from build123d import *

# Parameters (mm, degrees)
SKETCH1_W           = 20
SKETCH1_H           = 130
SKETCH1_R           = 2.5
BOSS_EXTRUDE1_DEPTH = 60
BOSS_EXTRUDE2_DEPTH = 130
CUT_EXTRUDE2_DEPTH  = 156.241746963
CUT_EXTRUDE3_DEPTH  = 25
SKETCH5_R           = 10
CUT_EXTRUDE4_DEPTH  = 147.694623422
SKETCH6_R           = 6
CUT_EXTRUDE8_DEPTH  = 55
SKETCH7_R           = 2.5
CUT_EXTRUDE9_DEPTH  = 5
SKETCH9_R           = 6
CUT_EXTRUDE10_DEPTH = 151.423561372


with BuildPart() as part:
    # Sketch1 → Boss-Extrude1 (new body)
    with BuildSketch(Plane.XY):
        with Locations((0, 65)):
            Rectangle(SKETCH1_W, SKETCH1_H)
        with Locations((0, 119.20647252)):
            Circle(SKETCH1_R, mode=Mode.SUBTRACT)
        with Locations((0, 68.70647252)):
            Circle(SKETCH1_R, mode=Mode.SUBTRACT)
    extrude(amount=BOSS_EXTRUDE1_DEPTH)

    # Sketch2 → Boss-Extrude2 (add)
    with BuildSketch(Plane(origin=(0, 130, 0), x_dir=(1, 0, 0), z_dir=(0, 1, 0))):
        Polygon((10, 0), (60, -50), (60, -60), (10, -60), align=None)
    extrude(amount=-BOSS_EXTRUDE2_DEPTH)

    # Sketch4 → Cut-Extrude2 (cut, through all)
    with BuildSketch(Plane(origin=(0, 0, 0), x_dir=(-1, 0, 0), z_dir=(0, 0, -1))):
        with BuildLine():
            ThreePointArc((-1.666666667, 129.066605492), (6.454972244, 126.844098678), (10, 119.20647252))
            Line((10, 119.20647252), (10, 130))
            Line((10, 130), (-10, 130))
            Line((-10, 130), (-10, 127.658015067))
            Line((-10, 127.658015067), (-1.666666667, 129.066605492))
        make_face()
        Polygon((-60, 130), (-60, 119.20647252), (-10, 127.658015067), (-10, 130), align=None)
    extrude(amount=-CUT_EXTRUDE2_DEPTH, mode=Mode.SUBTRACT)

    # Sketch4<5> → Cut-Extrude3 (cut)
    with BuildSketch(Plane(origin=(0, 0, 0), x_dir=(-1, 0, 0), z_dir=(0, 0, -1))):
        with BuildLine():
            Line((10, 0), (10, 68.70647252))
            ThreePointArc((10, 68.70647252), (6.454972244, 61.068846362), (-1.666666667, 58.846339548))
            Line((-1.666666667, 58.846339548), (-10, 60.254929973))
            Line((-10, 60.254929973), (-10, 0))
            Line((-10, 0), (10, 0))
        make_face()
        Polygon((-10, 60.254929973), (-60, 68.70647252), (-60, 0), (-10, 0), align=None)
    extrude(amount=-CUT_EXTRUDE3_DEPTH, mode=Mode.SUBTRACT)

    # Sketch5 → Cut-Extrude4 (cut, through all)
    with BuildSketch(Plane(origin=(0, 0, 25), x_dir=(-1, 0, 0), z_dir=(0, 0, -1))):
        with Locations((10, 0)):
            Circle(SKETCH5_R)
    extrude(amount=-CUT_EXTRUDE4_DEPTH, mode=Mode.SUBTRACT)

    # Sketch6 → Cut-Extrude8 (cut)
    with BuildSketch(Plane.XY.offset(60)):
        with Locations((0, 119.20647252)):
            Circle(SKETCH6_R)
        with Locations((0, 68.70647252)):
            Circle(SKETCH6_R)
    extrude(amount=-CUT_EXTRUDE8_DEPTH, mode=Mode.SUBTRACT)

    # Sketch7 → Cut-Extrude9 (cut)
    with BuildSketch(Plane.XZ):
        with Locations(Location((10, 50, 0), (0, 0, 270))):
            Circle(SKETCH7_R)
        with Locations(Location((40, 50, 0), (0, 0, 270))):
            Circle(SKETCH7_R)
        with Locations(Location((25, 35, 0), (0, 0, 270))):
            Circle(SKETCH7_R)
    extrude(amount=-CUT_EXTRUDE9_DEPTH, mode=Mode.SUBTRACT)

    # Sketch9 → Cut-Extrude10 (cut, through all)
    with BuildSketch(Plane.XZ.offset(-5)):
        with Locations(Location((10, 50, 0), (0, 0, 270))):
            Circle(SKETCH9_R)
        with Locations(Location((25, 35, 0), (0, 0, 270))):
            Circle(SKETCH9_R)
        with Locations(Location((40, 50, 0), (0, 0, 270))):
            Circle(SKETCH9_R)
    extrude(amount=-CUT_EXTRUDE10_DEPTH, mode=Mode.SUBTRACT)


solid = part.part
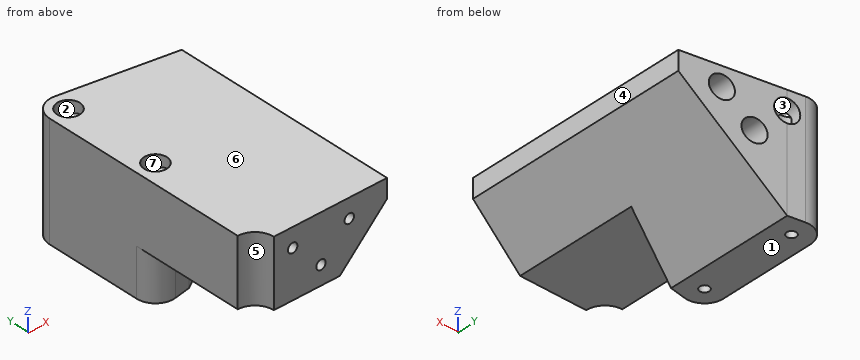
Source: CAD feature listing. Evaluate the final solid. Frame: model axes, mm. Face numbers are marked on the shaded views. A direction names the side the tool comes from. Give positions to 0.01 mm unless a question says otherwise; leave off trailing zeros. Order: outer loops, then holes, each group sorted by start corner. A loop starts at its lowest first (then second) coordinate and runs counter-clockwise, first axis right, second up. Notation, with made-up numbers: (83.5, 23.25) -> (112.5, 23.25) arc R3 ccw to (112.5, 28.25) -> close; hole circle Ø3 at (-34, -39). An arc over 180 degrees is marked (long way). Write item = value, one per line.
Q1. Cut plane C-C, the plane z = 27.5. Output: boundary loops of the cut face in (x, y), and give its area (3 significant figures).
Data:
outline = (-10, 10) arc R10 cw to (0, 0) -> (37.5, 0) -> (37.5, 123.01) -> (1.67, 129.07) arc R10 ccw to (-10, 119.21) -> close; hole circle Ø12 at (0, 68.71); hole circle Ø12 at (0, 119.21)
area = 5,700 mm^2
Q2. Pin query (flat end, axial travel): pin 1 (6.5 mm diameter, centred on x = 0, y = 68.71, fed in from +Z); pin 2 (6 mm diameter, centred on x = 25.5, z = 35, fed in from +Y); pin 3 (2 mm diameter, centred on x = 2, z = 19.5, fed in from -Y). Return the tip coordinate at first contact, or that it passes through.
Data:
pin_1 = 5
pin_2 = 5
pin_3 = 58.76
Q3. Cut plane D-D, the plane z = 35. Output: boundary loops of the cut face in (x, y).
Data:
outline = (-10, 10) arc R10 cw to (0, 0) -> (22.5, 0) -> (22.5, 5) -> (19, 5) -> (19, 126.14) -> (1.67, 129.07) arc R10 ccw to (-10, 119.21) -> close; (27.5, 0) -> (45, 0) -> (45, 121.74) -> (31, 124.11) -> (31, 5) -> (27.5, 5) -> close; hole circle Ø12 at (0, 68.71); hole circle Ø12 at (0, 119.21)
Q4. Material intervals for line 1 (Y direction, x = 0, z = 3.65); line 2 (X direction, y = 54, z = 50); line 3 (Y direction, x = -2, z = 38.5), sorted ascending. Write a range as from..to.
Data:
line_1 = 58.71..66.21, 71.21..116.71, 121.71..129.21
line_2 = -10..4, 16..34, 46..60
line_3 = 6..63.05, 74.36..113.55, 124.86..129
Q5. Cut plane B-B, the plane x = 25. Output: boundary loops of the cut face in (y, z), and give its area (3 significant figures).
Data:
outline = (0, 25) -> (62.79, 25) -> (62.79, 15) -> (125.12, 15) -> (125.12, 29) -> (5, 29) -> (5, 32.5) -> (0, 32.5) -> close; (0, 37.5) -> (5, 37.5) -> (5, 41) -> (125.12, 41) -> (125.12, 60) -> (0, 60) -> close
area = 3,540 mm^2
Q6. Cut plane A-A, the plane y = 34. Output: boundary loops of the cut face in (x, z), and give its area (3 significant figures).
Data:
outline = (-10, 25) -> (35, 25) -> (60, 50) -> (60, 60) -> (-10, 60) -> close; hole circle Ø12 at (10, 50); hole circle Ø12 at (25, 35); hole circle Ø12 at (40, 50)
area = 1,800 mm^2
Q7. Set-up query: the marked faces 1, 2 and 3. Return all of +Z, -Z, +X, -X, +Y, -Y with unobstructed straight access to the full face (end or side cutting, diameter ignored); none if empty.
Data:
face_1 = -Z, +X, -X, +Y, -Y
face_2 = +Z
face_3 = +Y
Q8. Pull-direction query (X, two-part tool) for the marked faces 4, 5, 6 and 7; classes: released by +X, released by -X, zero draft, split by the parting line, or undercut.
Data:
face_4 = released by +X
face_5 = released by -X
face_6 = zero draft
face_7 = undercut
